Build history of the part. All positions in model axes, mm. Face numbers are marked on the shaded views. A direction names the side the tool comes from. Round coordinates to 2 decimals unless told otherwise and drop trailing zeros. Write each loop counter-clockwise with the first axis right and the second up, starting at its lowest first coordinate (ties: lowest second). Pieces come first, ordered by that corner, then holes.
1) Which spindle directions (+Z, -Z, +X, -X, +Y, -Y) get a long thin tool onto all of the face, cutting with end or side? Do the marked faces 4 and 5. Say none if no direction does.
2) Saw through at A-A (z = 6.5). Write the cut outline in (x, y).
3) Saw through at B-B (y = 5.5). Write the cut outline in (x, z).
4) Saw through at C-C (x = 9.5). Write the cut outline in (y, z).
5) Flat gauge pins, fed straight in: pin 1 (1.5 mm diameter, centred on y = 0, z = 7, fed in from -X); pin 2 (1.5 mm diameter, centred on y = -12.5, z = 3, fed in from -X); pin 3 (2.5 mm diameter, centred on y = -4.5, z = 5, fed in from -X). Where does each tip first touch, or does it go through?
6) Pull direction Y, two halves, no side cores. Call the marked faces 1, 2 and 3: +Y half, -Y half, draft (parallel to the pull), parting line (faces both ways), or undercut.
7) Wall check: probe 1 along X at (y, z) = (1, 1.5); probe 2 along Z at (x, y) = (12, -9.5); probe 3 along Y at (x, z) = (-31.5, 1.5). Give the ranges that are in metal, low to high.
from build123d import *

# Parameters (mm, degrees)
SKETCH_W     = 100
SKETCH_H     = 60
PAD_DEPTH    = 10
FILLET_R     = 9
SKETCH001_W  = 80
SKETCH001_H  = 40
POCKET_DEPTH = 9


with BuildPart() as part:
    # Sketch → Pad (new body)
    with BuildSketch(Plane.XY):
        Rectangle(SKETCH_W, SKETCH_H)
    extrude(amount=PAD_DEPTH)

    # Fillet
    fillet_edges = [part.edges().sort_by_distance(p)[0] for p in [
        (0, -30, 10),
        (50, 0, 10),
        (0, 30, 10),
        (-50, 0, 10),
    ]]
    fillet(fillet_edges, radius=FILLET_R)

    # Sketch001 → Pocket (cut)
    with BuildSketch(Plane.XY.offset(10)):
        Rectangle(SKETCH001_W, SKETCH001_H)
    extrude(amount=-POCKET_DEPTH, mode=Mode.SUBTRACT)


solid = part.part
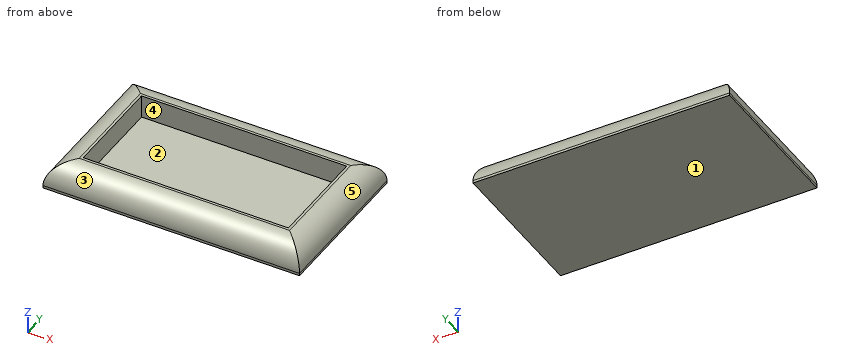
Evaluation:
1. face 4: +Z
1. face 5: +Z, +X, +Y, -Y
2. outline: (-48.12, -28.12) - (48.12, -28.12) - (48.12, 28.12) - (-48.12, 28.12) - close; hole (-40, -20) - (40, -20) - (40, 20) - (-40, 20) - close
3. outline: (-50, 0) - (50, 0) - (50, 1) arc R9 ccw to (41, 10) - (40, 10) - (40, 1) - (-40, 1) - (-40, 10) - (-41, 10) arc R9 ccw to (-50, 1) - close
4. outline: (-30, 0) - (30, 0) - (30, 1) arc R9 ccw to (21, 10) - (20, 10) - (20, 1) - (-20, 1) - (-20, 10) - (-21, 10) arc R9 ccw to (-30, 1) - close
5. pin 1: stops at x = -48.31
5. pin 2: stops at x = -49.91
5. pin 3: stops at x = -49.57
6. face 1: draft
6. face 2: undercut
6. face 3: -Y half
7. probe 1: x = -49.99 to -40, 40 to 49.99
7. probe 2: z = 0 to 1
7. probe 3: y = -29.99 to -20, 20 to 29.99
